The listing builds one solid part. Answer for the finished solid, in the listing's coordinates (mm). A direction names the side the tool comes from. Round coordinates to 2 decimals unless told otherwise and drop trailing zeros. Write each loop counter-clockwise with the first axis right and the second up, starting at its lowest first coordinate (ties: lowest second). Pieces come first, ordered by that corner, then holes. Notation, with made-up numbers: M 72.5,-38 L 127.5,-38 A16 cw 127.5,-24 Z; hole C 57,1.25 d7. An arc over 180 degrees is marked long. Put each result on its own line as item: value. Start each with the question number.
```python
from build123d import *

# Parameters (mm, degrees)
BOSS_EXTRUDE1_DEPTH = 8
CUT_EXTRUDE1_DEPTH  = 8
FILLET1_R           = 0.4
FILLET2_R           = 0.4
FILLET3_R           = 0.4
FILLET4_R           = 0.4
FILLET5_R           = 6.2
FILLET6_R           = 6.2
FILLET7_R           = 6.2
FILLET8_R           = 6.2
FILLET9_R           = 0.1
FILLET10_R          = 0.1
FILLET11_R          = 0.1
FILLET12_R          = 0.1
FILLET13_R          = 0.1
FILLET14_R          = 0.1
FILLET15_R          = 0.1
FILLET16_R          = 0.1
FILLET17_R          = 0.1
FILLET18_R          = 0.1
FILLET19_R          = 0.1
FILLET20_R          = 0.1
FILLET21_R          = 0.1
FILLET22_R          = 0.1
FILLET23_R          = 0.1
FILLET24_R          = 0.1


with BuildPart() as part:
    # Sketch1 → Boss-Extrude1 (new body)
    with BuildSketch(Plane.XY):
        with BuildLine():
            Line((-1.085, -1.085), (-1.085, -2.903924069))
            ThreePointArc((-1.085, -2.903924069), (0, -3.1), (1.085, -2.903924069))
            Line((1.085, -2.903924069), (1.085, -1.085))
            Line((1.085, -1.085), (2.903924069, -1.085))
            ThreePointArc((2.903924069, -1.085), (3.1, 0), (2.903924069, 1.085))
            Line((2.903924069, 1.085), (1.085, 1.085))
            Line((1.085, 1.085), (1.085, 2.903924069))
            ThreePointArc((1.085, 2.903924069), (0, 3.1), (-1.085, 2.903924069))
            Line((-1.085, 2.903924069), (-1.085, 1.085))
            Line((-1.085, 1.085), (-2.903924069, 1.085))
            ThreePointArc((-2.903924069, 1.085), (-3.1, 0), (-2.903924069, -1.085))
            Line((-2.903924069, -1.085), (-1.085, -1.085))
        make_face()
    extrude(amount=BOSS_EXTRUDE1_DEPTH)

    # Sketch2 → Cut-Extrude1 (cut)
    with BuildSketch(Plane.XY):
        with BuildLine():
            Line((0.84, -0.84), (2.248199279, -0.84))
            ThreePointArc((2.248199279, -0.84), (2.4, 0), (2.248199279, 0.84))
            Line((2.248199279, 0.84), (0.84, 0.84))
            Line((0.84, 0.84), (0.84, 2.248199279))
            ThreePointArc((0.84, 2.248199279), (0, 2.4), (-0.84, 2.248199279))
            Line((-0.84, 2.248199279), (-0.84, 0.84))
            Line((-0.84, 0.84), (-2.248199279, 0.84))
            ThreePointArc((-2.248199279, 0.84), (-2.4, 0), (-2.248199279, -0.84))
            Line((-2.248199279, -0.84), (-0.84, -0.84))
            Line((-0.84, -0.84), (-0.84, -2.248199279))
            ThreePointArc((-0.84, -2.248199279), (0, -2.4), (0.84, -2.248199279))
            Line((0.84, -2.248199279), (0.84, -0.84))
        make_face()
    extrude(amount=CUT_EXTRUDE1_DEPTH, mode=Mode.SUBTRACT)

    # Fillet1
    fillet1_edges = [part.edges().sort_by_distance(p)[0] for p in [
        (-0.84, 0.84, 4),
    ]]
    fillet(fillet1_edges, radius=FILLET1_R)

    # Fillet2
    fillet2_edges = [part.edges().sort_by_distance(p)[0] for p in [
        (0.84, 0.84, 4),
    ]]
    fillet(fillet2_edges, radius=FILLET2_R)

    # Fillet3
    fillet3_edges = [part.edges().sort_by_distance(p)[0] for p in [
        (0.84, -0.84, 4),
    ]]
    fillet(fillet3_edges, radius=FILLET3_R)

    # Fillet4
    fillet4_edges = [part.edges().sort_by_distance(p)[0] for p in [
        (-0.84, -0.84, 4),
    ]]
    fillet(fillet4_edges, radius=FILLET4_R)

    # Fillet5
    # the kernel refuses this fillet: 6.2 mm, written as the material it adds along each edge
    with BuildSketch(Plane(origin=(-1.085, 1.085, 0), x_dir=(-1, 0, 0), z_dir=(0, 0, 1))) as fillet5_piece_1:
        with BuildLine():
            CenterArc((5.198154004, -5.198154004), FILLET5_R, 123.027198012, 23.945603977)
            Line((0, -1.818924069), (0, 0))
            Line((0, 0), (1.818924069, 0))
        make_face()
    extrude(amount=8)

    # Fillet6
    # the kernel refuses this fillet: 6.2 mm, written as the material it adds along each edge
    with BuildSketch(Plane(origin=(-1.085, -1.085, 0), x_dir=(-1, 0, 0), z_dir=(0, 0, 1))) as fillet6_piece_1:
        with BuildLine():
            CenterArc((5.198154004, 5.198154004), FILLET6_R, 213.027198012, 23.945603977)
            Line((0, 1.818924069), (0, 0))
            Line((0, 0), (1.818924069, 0))
        make_face()
    extrude(amount=8)

    # Fillet7
    # the kernel refuses this fillet: 6.2 mm, written as the material it adds along each edge
    with BuildSketch(Plane(origin=(1.085, -1.085, 0), x_dir=(0, -1, 0), z_dir=(0, 0, 1))) as fillet7_piece_1:
        with BuildLine():
            CenterArc((5.198154004, 5.198154004), FILLET7_R, 213.027198012, 23.945603977)
            Line((0, 1.818924069), (0, 0))
            Line((0, 0), (1.818924069, 0))
        make_face()
    extrude(amount=8)

    # Fillet8
    # the kernel refuses this fillet: 6.2 mm, written as the material it adds along each edge
    with BuildSketch(Plane(origin=(1.085, 1.085, 0), x_dir=(1, 0, 0), z_dir=(0, 0, 1))) as fillet8_piece_1:
        with BuildLine():
            CenterArc((5.198154004, 5.198154004), FILLET8_R, 213.027198012, 23.945603977)
            Line((0, 1.818924069), (0, 0))
            Line((0, 0), (1.818924069, 0))
        make_face()
    extrude(amount=8)

    # Fillet9
    fillet9_edges = [part.edges().sort_by_distance(p)[0] for p in [
        (0.84, 2.248199279, 4),
    ]]
    fillet(fillet9_edges, radius=FILLET9_R)

    # Fillet10
    fillet10_edges = [part.edges().sort_by_distance(p)[0] for p in [
        (1.085, 2.903924069, 4),
    ]]
    fillet(fillet10_edges, radius=FILLET10_R)

    # Fillet11
    fillet11_edges = [part.edges().sort_by_distance(p)[0] for p in [
        (-1.085, 2.903924069, 4),
    ]]
    fillet(fillet11_edges, radius=FILLET11_R)

    # Fillet12
    fillet12_edges = [part.edges().sort_by_distance(p)[0] for p in [
        (-2.903924069, 1.085, 4),
    ]]
    fillet(fillet12_edges, radius=FILLET12_R)

    # Fillet13
    fillet13_edges = [part.edges().sort_by_distance(p)[0] for p in [
        (-2.903924069, -1.085, 4),
    ]]
    fillet(fillet13_edges, radius=FILLET13_R)

    # Fillet14
    fillet14_edges = [part.edges().sort_by_distance(p)[0] for p in [
        (-1.085, -2.903924069, 4),
    ]]
    fillet(fillet14_edges, radius=FILLET14_R)

    # Fillet15
    fillet15_edges = [part.edges().sort_by_distance(p)[0] for p in [
        (1.085, -2.903924069, 4),
    ]]
    fillet(fillet15_edges, radius=FILLET15_R)

    # Fillet16
    fillet16_edges = [part.edges().sort_by_distance(p)[0] for p in [
        (2.903924069, -1.085, 4),
    ]]
    fillet(fillet16_edges, radius=FILLET16_R)

    # Fillet17
    fillet17_edges = [part.edges().sort_by_distance(p)[0] for p in [
        (2.903924069, 1.085, 4),
    ]]
    fillet(fillet17_edges, radius=FILLET17_R)

    # Fillet18
    fillet18_edges = [part.edges().sort_by_distance(p)[0] for p in [
        (0.84, -2.248199279, 4),
    ]]
    fillet(fillet18_edges, radius=FILLET18_R)

    # Fillet19
    fillet19_edges = [part.edges().sort_by_distance(p)[0] for p in [
        (-0.84, -2.248199279, 4),
    ]]
    fillet(fillet19_edges, radius=FILLET19_R)

    # Fillet20
    fillet20_edges = [part.edges().sort_by_distance(p)[0] for p in [
        (-2.248199279, 0.84, 4),
    ]]
    fillet(fillet20_edges, radius=FILLET20_R)

    # Fillet21
    fillet21_edges = [part.edges().sort_by_distance(p)[0] for p in [
        (-2.248199279, -0.84, 4),
    ]]
    fillet(fillet21_edges, radius=FILLET21_R)

    # Fillet22
    fillet22_edges = [part.edges().sort_by_distance(p)[0] for p in [
        (-0.84, 2.248199279, 4),
    ]]
    fillet(fillet22_edges, radius=FILLET22_R)

    # Fillet23
    fillet23_edges = [part.edges().sort_by_distance(p)[0] for p in [
        (2.248199279, -0.84, 4),
    ]]
    fillet(fillet23_edges, radius=FILLET23_R)

    # Fillet24
    fillet24_edges = [part.edges().sort_by_distance(p)[0] for p in [
        (2.248199279, 0.84, 4),
    ]]
    fillet(fillet24_edges, radius=FILLET24_R)


solid = part.part
```
Item 1: Consider line 1 along Y through (x, z) = (0.75, 3.75); line 2 along X through (y, z) = (1, 1.5); line 3 along Y through (x, z) = (2, 4.75). Determine where each line is inside the solid, lowest interval first. Write a range as [from, to].
Item 2: Section C-C (y = 2.75) is taken. Give the vertices of the cut face in (x, z).
Item 3: Flat-ended cylindrical pins translate along their axes: pin 1 (0.5 mm diameter, centred on y = 1.5, z = 6, fed in from +X); pin 2 (1 mm diameter, centred on y = -1.5, z = 4, fed in from -X); pin 3 (0.5 mm diameter, centred on x = 2, z = 3, fed in from -Y). Find the tip coordinate at first contact, or state that the pin passes through.
Item 4: Which of the six approach directions +Z, -Z, +X, -X, +Y, -Y give full straight-line access (tool end or side, diameter ignored) to faces 1 (the cylindrical face through (-2.4, 0, 3.9)), 2 (the cylindrical face through (0, 3.1, 3.9))?
Item 5: Section A-A (x = -0.5) is taken. Give the vertices of the cut face in (y, z).
Item 6: Determine the mould class of faces 3 (the cylindrical face through (1.9, 1.9, 3.9)), 4 (the flat face through (0.84, -2, 4)), 5 (the cylindrical face through (-3.1, 0, 3.9)), 6 (the flat face through (1.2, 1.2, 8)) for opening direction Y: released by +Y, released by -Y, zero draft, split by the parting line, or undercut.
Output values:
1. line 1: y = [-3.01, -2.28], [2.28, 3.01]
1. line 2: x = [-2.93, -0.92], [0.92, 2.93]
1. line 3: y = [-1.8, -0.84], [0.84, 1.8]
2. outline: M -1.19,0 L 1.19,0 L 1.19,8 L -1.19,8 Z
3. pin 1: stops at x = 2.66
3. pin 2: stops at x = -2.93
3. pin 3: stops at y = -2.05
4. face 1: +Z, -Z
4. face 2: +Z, -Z, +Y
5. outline: M -3.06,0 L -2.35,0 L -2.35,8 L -3.06,8 Z; M 2.35,0 L 3.06,0 L 3.06,8 L 2.35,8 Z
6. face 3: released by +Y
6. face 4: undercut
6. face 5: split by the parting line
6. face 6: zero draft
